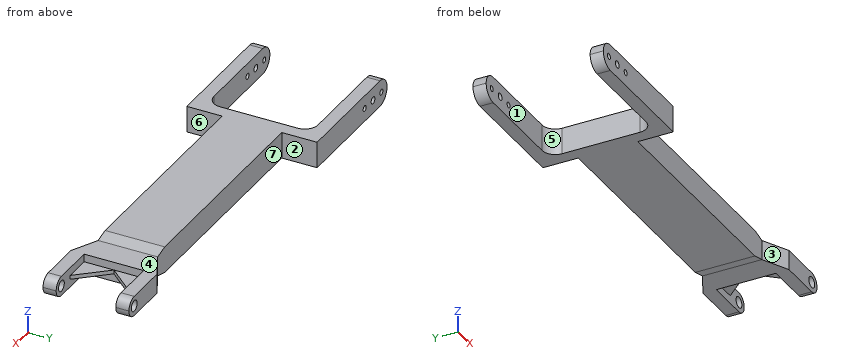
from build123d import *

# Parameters (mm, degrees)
SKETCH_2_W               = 187.5
SKETCH_2_H               = 45.3
EXTRUDE_1_DEPTH          = 10
EXTRUDE_2_DEPTH          = 7.5
CHAMFER_1_SIZE           = 20
CHAMFER_1_SIZE_2         = 5
CHAMFER_2_SIZE           = 5
CHAMFER_2_SIZE_2         = 20
SKETCH_7_W               = 40
SKETCH_7_H               = 10
EXTRUDE_6_DEPTH          = 15
SKETCH_7_3_W             = 40
SKETCH_7_3_H             = 10
CUT_EXTRUDE_3_DEPTH      = 15
EXTRUDE_7_DEPTH          = 1.5
CUT_EXTRUDE_1_DEPTH      = 314.699298692
CUT_EXTRUDE_2_DEPTH      = 307.287238552
CUT_EXTRUDE_2_DEPTH_BACK = 307.287238552
FILLET_1_R               = 10


with BuildPart() as part:
    # 草图2 → 凸台-拉伸1 (new, symmetric)
    with BuildSketch(Plane.XY):
        with Locations((-103.75, 0)):
            Rectangle(SKETCH_2_W, SKETCH_2_H)
        Polygon((-297.5, 49.5), (-297.5, 39.5), (-207.5, 39.5), (-207.5, -39.5), (-297.5, -39.5), (-297.5, -49.5), (-197.5, -49.5), (-197.5, 49.5), align=None)
    extrude(amount=EXTRUDE_1_DEPTH, both=True)

    # 草图2<3> → 凸台-拉伸2 (add, symmetric)
    with BuildSketch(Plane.XY):
        Polygon((40, -22.65), (40, -12.65), (0, -12.65), (0, 12.65), (40, 12.65), (40, 22.65), (-10, 22.65), (-10, -22.65), align=None)
    extrude(amount=EXTRUDE_2_DEPTH, both=True)

    # 倒角1
    # the kernel refuses this chamfer: 20, 5 mm, written as the material it takes off along each edge
    with BuildSketch(Plane(origin=(-10, -74.592549995, 10), x_dir=(-0.9999563942249224, 0, 0.00933861064031752), z_dir=(0, 1, 0))) as chamfer_1_piece_1_section:
        Polygon((CHAMFER_1_SIZE * 0.999956394225, -CHAMFER_1_SIZE * 0.00933861064032), (-CHAMFER_1_SIZE_2 * 0.00933861064032, -CHAMFER_1_SIZE_2 * 0.999956394225), (0, 0), align=None)
    chamfer_1_piece_1 = extrude(amount=149.185099991, mode=Mode.PRIVATE)
    chamfer_1_piece_1 = split(chamfer_1_piece_1, bisect_by=Plane(origin=(-18.245866107, 0, 7.5), z_dir=(0, 0, 1)), keep=Keep.TOP, mode=Mode.PRIVATE)
    add(chamfer_1_piece_1, mode=Mode.SUBTRACT)

    # 倒角2
    # the kernel refuses this chamfer: 20, 5 mm, written as the material it takes off along each edge
    with BuildSketch(Plane(origin=(-10, -74.592549995, -10), x_dir=(0.14778356633657133, 0, 0.9890197255468893), z_dir=(0, 1, 0))) as chamfer_2_piece_1_section:
        Polygon((CHAMFER_2_SIZE * 0.989019725547, -CHAMFER_2_SIZE * 0.147783566337), (-CHAMFER_2_SIZE_2 * 0.147783566337, -CHAMFER_2_SIZE_2 * 0.989019725547), (0, 0), align=None)
    chamfer_2_piece_1 = extrude(amount=149.185099991, mode=Mode.PRIVATE)
    chamfer_2_piece_1 = split(chamfer_2_piece_1, bisect_by=Plane(origin=(-18.245866107, 0, -7.5), z_dir=(0, 0, -1)), keep=Keep.TOP, mode=Mode.PRIVATE)
    add(chamfer_2_piece_1, mode=Mode.SUBTRACT)

    # 草图7 → 凸台-拉伸6 (add)
    with BuildSketch(Plane.XY.offset(7.5)):
        Polygon((0, 22.65), (0, 32.65), (-20, 22.65), align=None)
        with Locations((20, 27.65)):
            Rectangle(SKETCH_7_W, SKETCH_7_H)
        Polygon((40, -32.65), (0, -32.65), (-20, -22.65), (40, -22.65), align=None)
    extrude(amount=-EXTRUDE_6_DEPTH)

    # 草图7<3> → 切除-拉伸3 (cut)
    with BuildSketch(Plane.XY.offset(7.5)):
        with Locations((20, 17.65)):
            Rectangle(SKETCH_7_3_W, SKETCH_7_3_H)
        with Locations((20, -17.65)):
            Rectangle(SKETCH_7_3_W, SKETCH_7_3_H)
    extrude(amount=-CUT_EXTRUDE_3_DEPTH, mode=Mode.SUBTRACT)

    # 草图8 → 凸台-拉伸7 (add, symmetric)
    with BuildSketch(Plane.XY):
        Polygon((0, 22.65), (0, 0), (20, 22.65), align=None)
        Polygon((20, -22.65), (0, 0), (0, -22.65), align=None)
    extrude(amount=EXTRUDE_7_DEPTH, both=True)

    # 草图3 → 切除-拉伸1 (cut, through all)
    with BuildSketch(Plane(origin=(0, 49.5, 0), x_dir=(1, 0, 0), z_dir=(0, 1, 0))):
        with BuildLine():
            ThreePointArc((-297.5, 0), (-294.571067812, 7.071067812), (-287.5, 10))
            Line((-287.5, 10), (-297.5, 10))
            Line((-297.5, 10), (-297.5, 0))
        make_face()
        with BuildLine():
            Line((-297.5, -10), (-287.5, -10))
            ThreePointArc((-287.5, -10), (-294.571067812, -7.071067812), (-297.5, 0))
            Line((-297.5, 0), (-297.5, -10))
        make_face()
        with BuildLine():
            ThreePointArc((-291.65, 0), (-289.5, -2.15), (-287.35, 0))
            Line((-287.35, 0), (-291.65, 0))
        make_face()
        with BuildLine():
            Line((-291.65, 0), (-287.35, 0))
            ThreePointArc((-287.35, 0), (-289.5, 2.15), (-291.65, 0))
        make_face()
        with BuildLine():
            ThreePointArc((-280.15, 0), (-277.5, -2.65), (-274.85, 0))
            Line((-274.85, 0), (-280.15, 0))
        make_face()
        with BuildLine():
            Line((-280.15, 0), (-274.85, 0))
            ThreePointArc((-274.85, 0), (-277.5, 2.65), (-280.15, 0))
        make_face()
        with BuildLine():
            ThreePointArc((-267.65, 0), (-265.5, -2.15), (-263.35, 0))
            Line((-263.35, 0), (-267.65, 0))
        make_face()
        with BuildLine():
            Line((-267.65, 0), (-263.35, 0))
            ThreePointArc((-263.35, 0), (-265.5, 2.15), (-267.65, 0))
        make_face()
    extrude(amount=-CUT_EXTRUDE_1_DEPTH, mode=Mode.SUBTRACT)

    # 草图4 → 切除-拉伸2 (cut, two sides: drawn at the far end of the back side and taken through both)
    with BuildSketch(Plane(origin=(0, 22.65, 0), x_dir=(1, 0, 0), z_dir=(0, 1, 0)).offset(-CUT_EXTRUDE_2_DEPTH_BACK)):
        with BuildLine():
            Line((28.35, 0), (36.65, 0))
            ThreePointArc((36.65, 0), (32.5, 4.15), (28.35, 0))
        make_face()
        with BuildLine():
            ThreePointArc((28.35, 0), (32.5, -4.15), (36.65, 0))
            Line((36.65, 0), (28.35, 0))
        make_face()
        with BuildLine():
            ThreePointArc((32.5, 7.5), (37.803300859, 5.303300859), (40, 0))
            Line((40, 0), (40, 7.5))
            Line((40, 7.5), (32.5, 7.5))
        make_face()
        with BuildLine():
            Line((40, -7.5), (40, 0))
            ThreePointArc((40, 0), (37.803300859, -5.303300859), (32.5, -7.5))
            Line((32.5, -7.5), (40, -7.5))
        make_face()
    extrude(amount=CUT_EXTRUDE_2_DEPTH + CUT_EXTRUDE_2_DEPTH_BACK, mode=Mode.SUBTRACT)

    # 圆角1
    fillet_1_edges = [part.edges().sort_by_distance(p)[0] for p in [
        (-207.5, -39.5, 0),
        (-207.5, 39.5, 0),
    ]]
    fillet(fillet_1_edges, radius=FILLET_1_R)


solid = part.part
Check sheet for the modelled part. Datum: model origin and axes. Units: mm. Face numbers are marked on the shaded views. A direction names the side the tool comes from. Give positions to 0.01 mm unless a question says otherwise; leave off trailing zeros. Write each loop counter-clockwise with the first axis right and the second up, starting at its lowest first coordinate (ties: lowest second). Pieces come first, ordered by that corner, then holes. Notation, with made-up numbers: (82, 39) -> (136, 39) arc R23 ccw to (136, 53) -> close; hole circle Ø3 at (70.25, 86). An arc over 180 degrees is marked (long way). One line per item, written item: value. Start each with the question number.
Item 1: Section check D-D on y = -5. Record the cut outline in (x, z), then the cut area to 3 significant figures.
Item 2: Gauge pin test, flat ends, axial feed: pin 1 (7.5 mm diameter, centred on x = 25.5, z = -3, fed in from +Y); pin 2 (4 mm diameter, centred on x = -26.5, z = 3, fed in from +Y); pin 3 (10 mm diameter, centred on x = -112, z = -5.5, fed in from -Y). Record the tip position at first contact, or that the pin passes through.
Item 3: Material ranges on probe 1 along Y at (x, z) = (2.5, -5.25); probe 2 along Z at (x, y) = (-265.5, -44.5), recorded low to high. Write a range as from..to.
Item 4: Tool access check on the marked faces 1, 2 and 3. Record the directions out of +Z, -Z, +X, -X, +Y, -Y that give a thin tool (end or side, any length) a straight path to the whole face; none if there is none.
Item 5: Section check B-B on x = -226. Record the cut outline in (y, z).
Item 6: Section check A-A on y = 26.5. Record the cut outline in (x, z).
Item 7: Section check C-C on y = 43. Record the cut outline in (x, z), then the cut area to 3 significant figures.
Item 8: Draft check along X on the marked faces 4, 5, 6 and 7. Enter one of: +X half, -X half, draft (parallel to the pull), parting line (faces both ways), or undercut.
Results list:
1. outline: (-207.5, -10) -> (-30, -10) -> (-20, -7.5) -> (0, -7.5) -> (0, -1.5) -> (4.42, -1.5) -> (4.42, 1.5) -> (0, 1.5) -> (0, 7.5) -> (-20, 7.5) -> (-30, 10) -> (-207.5, 10) -> close
1. area: 4,040 mm²
2. pin 1: y = 32.65
2. pin 2: y = 22.65
2. pin 3: y = -22.65
3. probe 1: -32.65..-22.65, 22.65..32.65
3. probe 2: -10..-2.15, 2.15..10
4. face 1: +Z, -Z, -X
4. face 2: +Z, -Z, +Y
4. face 3: +Z, -Z, -Y
5. outline: (-49.5, -10) -> (-39.5, -10) -> (-39.5, 10) -> (-49.5, 10) -> close; (39.5, -10) -> (49.5, -10) -> (49.5, 10) -> (39.5, 10) -> close
6. outline: (-207.5, -10) -> (-197.5, -10) -> (-197.5, 10) -> (-207.5, 10) -> close; (-12.3, -7.5) -> (32.5, -7.5) arc R7.5 ccw to (32.5, 7.5) -> (-12.3, 7.5) -> close; hole circle Ø8.3 at (32.5, 0)
7. outline: (-287.5, -10) -> (-197.5, -10) -> (-197.5, 10) -> (-287.5, 10) arc R10 ccw to start; hole circle Ø4.3 at (-289.5, 0); hole circle Ø5.3 at (-277.5, 0); hole circle Ø4.3 at (-265.5, 0)
7. area: 1,910 mm²
8. face 4: draft
8. face 5: -X half
8. face 6: undercut
8. face 7: undercut
